from build123d import *

# Parameters (mm, degrees)
SKETCH1_W           = 127
SKETCH1_H           = 76.2
BASE_EXTRUDE_DEPTH  = 12.7
BOSS_EXTRUDE2_DEPTH = 25.4
SKETCH4_R           = 6.35
CUT_EXTRUDE1_DEPTH  = 143.275747443
SKETCH5_R           = 12.7
CUT_EXTRUDE2_DEPTH  = 87.702150572


with BuildPart() as part:
    # Sketch1 → Base-Extrude (new body)
    with BuildSketch(Plane(origin=(0, 0, 0), x_dir=(1, 0, 0), z_dir=(0, 1, 0))):
        Rectangle(SKETCH1_W, SKETCH1_H)
    extrude(amount=BASE_EXTRUDE_DEPTH)

    # Sketch3 → Boss-Extrude2 (add, symmetric)
    with BuildSketch(Plane(origin=(0, 0, 0), x_dir=(0, 0, -1), z_dir=(1, 0, 0))):
        Polygon((-25.4, 12.7), (24.442365435, 47.6), (38.1, 47.6), (38.1, 12.7), align=None)
    extrude(amount=BOSS_EXTRUDE2_DEPTH, both=True)

    # Sketch4 → Cut-Extrude1 (cut, through all)
    with BuildSketch(Plane(origin=(65.699574279, 12.7, 10.189215324), x_dir=(-1, 0, 0), z_dir=(0, 1, 0))):
        with Locations(Location((14.899574279, -22.889215324, 0), (0, 0, 90))):
            Circle(SKETCH4_R)
        with Locations(Location((116.499574279, 2.510784676, 0), (0, 0, 90))):
            Circle(SKETCH4_R)
    extrude(amount=-CUT_EXTRUDE1_DEPTH, mode=Mode.SUBTRACT)

    # Sketch5 → Cut-Extrude2 (cut, through all)
    with BuildSketch(Plane(origin=(0, 20.455924194, 14.323392322), x_dir=(-1, 0, 0), z_dir=(0, 0.8191520442889948, 0.5735764363510417))):
        with Locations(Location((6.3, -9.224251984, 0), (0, 0, 90))):
            Circle(SKETCH5_R)
    extrude(amount=-CUT_EXTRUDE2_DEPTH, mode=Mode.SUBTRACT)


solid = part.part
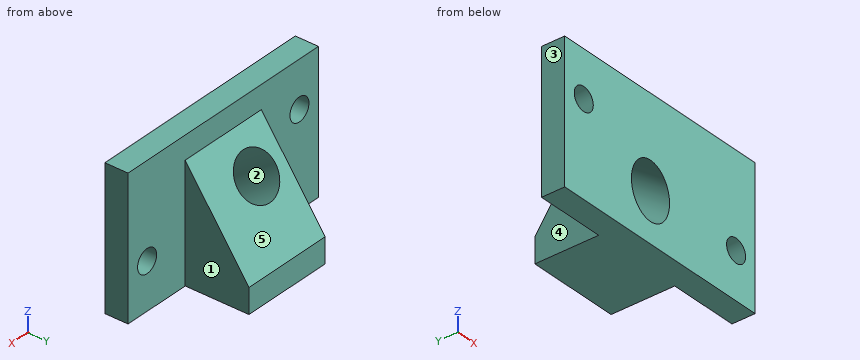
Source: CAD feature listing. Evaluate the final solid. Frame: model axes, mm. Face numbers are marked on the shaded views. A direction names the side the tool comes from. Round coordinates to 2 decimals unless told otherwise and drop trailing zeros. Loops run counter-clockwise (first coordinate to the right, second up) from the corner with the lowest first, then second, coordinate; pieces in that order, holes last.
Q1. Ray query, line 1 (X direction, y = 21, z = 2.5); line 2 (X direction, y = 3.75, z = -12.7); line 3 (Y direction, x = -53, z = 1). Return the intervals inside material, ascending.
Q2. Section A-A, the plane x = 50.8. Return loops of the section in (y, z).
Q3. Section D-D, the plane x = 5. Return loops of the section in (y, z).
Q4. Section B-B, the plane z = -31.5. Return loops of the section in (x, y), plus the area to 3 significant figures.
Q5. First-contact query: P1, Ø1, axis at x = -17.5, z = 21.5, coming from the +Y side; P2, Ø2, axis at x = 0.5, z = -7.5, coming from the +Y side; P3, Ø17.5, axis at y = 23, z = -11, coming from the -X side. Flat tips, straight axial feed; report the tip coordinate or a pass-through.
Q6. Section C-C, the plane x = -20.5. Return loops of the section in (y, z).
Q7. Access query for the marked faces 4 and 5. Directions: +Z, -Z, +X, -X, +Y, -Y. A direction counts if a zero-diameter tool reaches every point of the face in a straight line with its end or side. Return the directions, or none.
Q8. Mould query, pull axis X, two halves, no side actions, for the marked faces 1, 2 and 3. Classes: pulls with the +X half, pulls with the -X half, needs draft (parallel to the pull), parting line crosses it, or undercut.
Solutions:
1. line 1: x = -25.4 to -18.98, 6.38 to 25.4
1. line 2: x = -63.5 to -18.56, 5.96 to 44.45, 57.15 to 63.5
1. line 3: y = 0 to 12.7
2. outline: (0, -38.1) - (12.7, -38.1) - (12.7, -19.05) - (0, -19.05) - close; (0, -6.35) - (12.7, -6.35) - (12.7, 38.1) - (0, 38.1) - close
3. outline: (0, -38.1) - (47.6, -38.1) - (47.6, -24.44) - (29.07, 2.02) - (0, -18.34) - close; (0, -4.18) - (22.42, 11.52) - (12.7, 25.4) - (12.7, 38.1) - (0, 38.1) - close
4. outline: (-63.5, 0) - (63.5, 0) - (63.5, 12.7) - (25.4, 12.7) - (25.4, 47.6) - (-25.4, 47.6) - (-25.4, 12.7) - (-63.5, 12.7) - close
4. area: 3,390 mm2
5. P1: stops at y = 15.78
5. P2: stops at y = 36.44
5. P3: stops at x = -25.4
6. outline: (0, -38.1) - (47.6, -38.1) - (47.6, -24.44) - (12.7, 25.4) - (12.7, 38.1) - (0, 38.1) - close
7. face 4: +Z, -Z, -X, +Y
7. face 5: +Z, +X, -X, +Y
8. face 1: pulls with the +X half
8. face 2: undercut
8. face 3: pulls with the -X half
